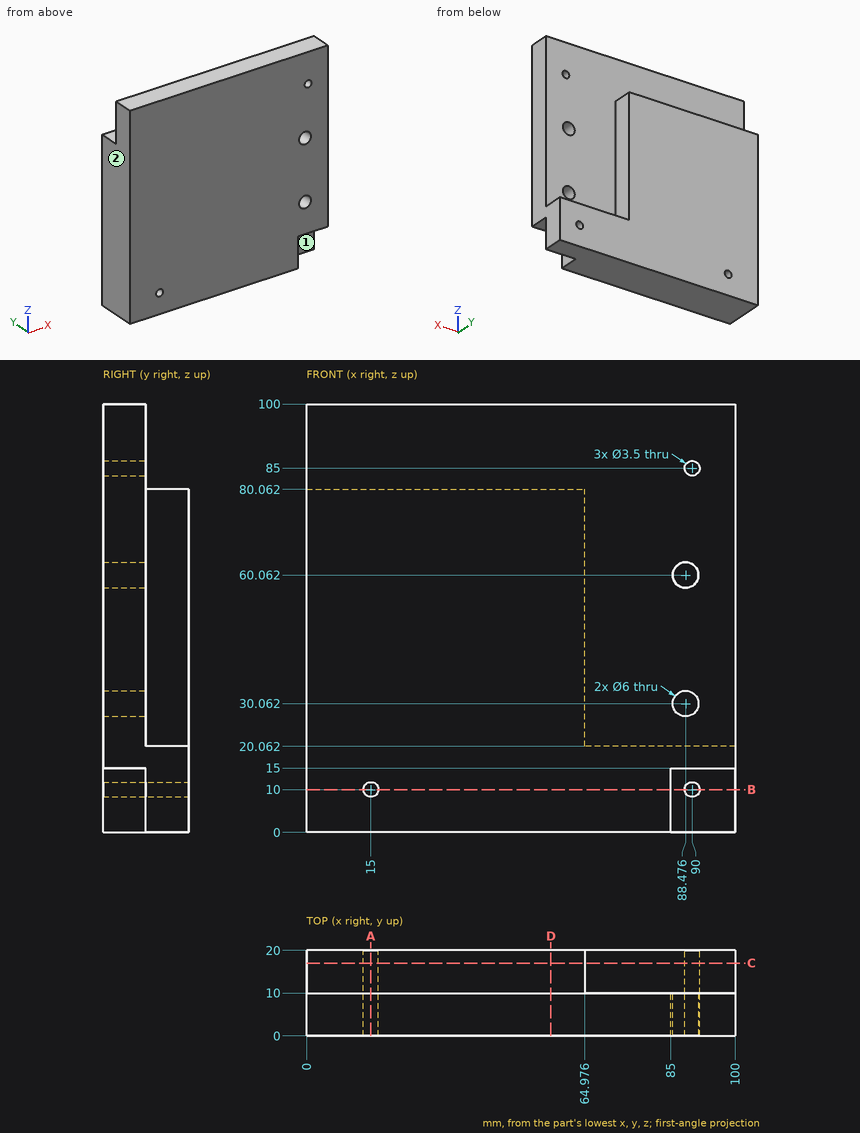
Answer from the drawing. Dimensions are ordinates in mm from the lowest x, y and z of the part. A direction names the side the tool comes from. Round coordinates to 2 decimals unless told otherwise and drop trailing zeros. Write each loop counter-clockwise with the first axis right and the second up, starting at its lowest first coordinate (ties: lowest second). Pieces come first, ordered by that corner, then holes. Notation, with made-up numbers: (21, 38) - (40, 38) arc R27 cw to (40, 55) - close; hole circle Ø1 at (51, 61.5). An arc over 180 degrees is marked (long way). Use a Markdown table: item, result.
(1) Which of the six approach directions +Z, -Z, +X, -X, +Y, -Y give full straight-line access (tool end or side, diameter ignored) to the marked faces 1 and 2?
Reported:
| item | result |
|---|---|
| face 1 | -Z, +X, -Y |
| face 2 | +Z, -Z, -X, +Y, -Y |
(2) The part is cut by section D-D (x = 57). Write down the section's boundary in (y, z), then the cut area to 3 significant figures.
Reported:
| item | result |
|---|---|
| outline | (0, 0) - (20, 0) - (20, 80.06) - (10, 80.06) - (10, 100) - (0, 100) - close |
| area | 1,800 mm2 |
(3) The part is cut by section B-B (z = 10). Write down the section's boundary in (x, y), then the cut area to 4 significant figures.
Reported:
| item | result |
|---|---|
| outline | (0, 0) - (13.25, 0) - (13.25, 20) - (0, 20) - close; (16.75, 0) - (85, 0) - (85, 10) - (88.25, 10) - (88.25, 20) - (16.75, 20) - close; (91.75, 10) - (100, 10) - (100, 20) - (91.75, 20) - close |
| area | 1,745 mm2 |
(4) The part is cut by section A-A (x = 15). Write down the section's boundary in (y, z), then the cut area to 3 significant figures.
Reported:
| item | result |
|---|---|
| outline | (0, 0) - (20, 0) - (20, 8.25) - (0, 8.25) - close; (0, 11.75) - (20, 11.75) - (20, 80.06) - (10, 80.06) - (10, 100) - (0, 100) - close |
| area | 1,730 mm2 |
(5) The part is cut by section C-C (y = 17). Write down the section's boundary in (x, z), then the cut area to 3 significant figures.
Reported:
| item | result |
|---|---|
| outline | (0, 0) - (100, 0) - (100, 20.06) - (64.98, 20.06) - (64.98, 80.06) - (0, 80.06) - close; hole circle Ø3.5 at (15, 10); hole circle Ø3.5 at (90, 10) |
| area | 5,890 mm2 |
(6) Straight lines are drawn through the part: line 1 along X through (y, z) = (13.5, 10); line 2 along X through (y, z) = (14.5, 9) (1 decimal); line 3 along Z through (x, y) = (15, 12). For each, find the intervals that lie inside material, in ascending order. Write a range as [from, to].
Reported:
| item | result |
|---|---|
| line 1 | [0, 13.25], [16.75, 88.25], [91.75, 100] |
| line 2 | [0, 13.6], [16.4, 88.6], [91.4, 100] |
| line 3 | [0, 8.25], [11.75, 80.06] |
(7) Each of these flat-tipped pins is pushed along its axis until it touches: pin 1 Ø3 at (x, y) = (90.5, 17) entering from +Z; pin 2 Ø7.5 at (x, z) = (91, 4.5) entering from -Y; pin 3 Ø11 at (x, y) = (33.5, 16) entering from +Z. Where does it stop, or does it pass through?
Reported:
| item | result |
|---|---|
| pin 1 | z = 20.06 |
| pin 2 | y = 10 |
| pin 3 | z = 80.06 |
